from build123d import *

# Parameters (mm, degrees)
BOSS_EXTRUDE1_DEPTH         = 50.8
SKETCH2_R                   = 3.2639
F_1_4_CLEARNACE_HOLES_DEPTH = 9.4996
CUT_EXTRUDE2_REACH          = 75.836
SKETCH3_R                   = 4.7625
SKETCH4_R                   = 4.7625
F_3_8_HEAD_DEPTH            = 5.08


with BuildPart() as part:
    # Sketch1 → Boss-Extrude1 (new body)
    with BuildSketch(Plane(origin=(0, 0, 0), x_dir=(0, 0, -1), z_dir=(1, 0, 0))):
        Polygon((41.796907359, 27.1145), (9.4996, 27.1145), (9.4996, 6.4135), (41.796907359, 6.4135), (41.796907359, 0), (0, 0), (0, 33.528), (41.796907359, 33.528), align=None)
    extrude(amount=BOSS_EXTRUDE1_DEPTH)

    # Sketch2 → 1/4 Clearnace Holes (cut)
    with BuildSketch(Plane(origin=(0, 0, -9.4996), x_dir=(-1, 0, 0), z_dir=(0, 0, -1))):
        with Locations(Location((-38.1, 16.764, 0), (0, 0, 90))):
            Circle(SKETCH2_R)
        with Locations(Location((-12.7, 16.764, 0), (0, 0, 90))):
            Circle(SKETCH2_R)
    extrude(amount=-F_1_4_CLEARNACE_HOLES_DEPTH, mode=Mode.SUBTRACT)

    # Cut-Extrude2: up to this face of the body (flat: up to its plane)
    cut_extrude2_end = Plane(part.part.faces().sort_by_distance((25.4, 33.528, -20.898453679))[0])
    # Sketch3 → Cut-Extrude2 (cut, up to the picked face)
    with BuildSketch(Plane.XZ, mode=Mode.PRIVATE) as cut_extrude2_sk1:
        with Locations(Location((25.4, -25.286907359, 0), (0, 0, 270))):
            Circle(SKETCH3_R)
    cut_extrude2_tool1 = split(extrude(cut_extrude2_sk1.sketch, amount=-CUT_EXTRUDE2_REACH, mode=Mode.PRIVATE), bisect_by=cut_extrude2_end, keep=Keep.BOTH, mode=Mode.PRIVATE)
    # Sketch3 → Cut-Extrude2 (cut, up to the picked face)
    with BuildSketch(Plane.XZ, mode=Mode.PRIVATE) as cut_extrude2_sk2:
        with BuildLine():
            Line((0, -12.7), (13.468510474, -33.146437494))
            ThreePointArc((13.468510474, -33.146437494), (25.4, -39.574407359), (37.331489526, -33.146437494))
            Line((37.331489526, -33.146437494), (50.8, -12.7))
            Line((50.8, -12.7), (50.8, -41.796907359))
            Line((50.8, -41.796907359), (0, -41.796907359))
            Line((0, -41.796907359), (0, -12.7))
        make_face()
    cut_extrude2_tool2 = split(extrude(cut_extrude2_sk2.sketch, amount=-CUT_EXTRUDE2_REACH, mode=Mode.PRIVATE), bisect_by=cut_extrude2_end, keep=Keep.BOTH, mode=Mode.PRIVATE)
    add(cut_extrude2_tool1.solids().sort_by(Axis((25.4, 0, -25.286907), (0, 1, 0)))[0], mode=Mode.SUBTRACT)
    add(cut_extrude2_tool2.solids().sort_by(Axis((6.245364, 0, -23.245262), (0, 1, 0)))[0], mode=Mode.SUBTRACT)

    # Sketch4 → 3/8 Head (cut)
    with BuildSketch(Plane(origin=(0, 0, -9.4996), x_dir=(-1, 0, 0), z_dir=(0, 0, -1))):
        with Locations(Location((-12.7, 16.764, 0), (0, 0, 90))):
            Circle(SKETCH4_R)
        with Locations(Location((-38.1, 16.764, 0), (0, 0, 90))):
            Circle(SKETCH4_R)
    extrude(amount=-F_3_8_HEAD_DEPTH, mode=Mode.SUBTRACT)


solid = part.part
Could you check a few things on this model? Use its own coordinates, in mm. A direction names the side the tool comes from. Coordinates: 2 decimals unless noted, no trailing zeros. Order: outer loops, then holes, each group sorted by start corner. A loop starts at its lowest first (then second) coordinate and runs counter-clockwise, first axis right, second up. Notation, with made-up numbers: (47, -30.75) - (58, -30.75) arc R19 ccw to (58, -21.75) - close; hole circle Ø2 at (36.25, 42.5). An arc over 180 degrees is marked (long way). Answer in a Markdown table with one row per item. Add a question column.
(1) If we section it at A-A, the plane x = 25.4: Please give me the cut outline in (y, z), then the cut area to 3 significant figures.
(2) Will these pins go through, and if not, where does the flat tip stop? pin 1 (3 mm diameter, centred on x = 38.5, y = 16.5, fed in from -Z); pin 2 (6 mm diameter, centred on x = 20.5, y = 13, fed in from -Z); pin 3 (10 mm diameter, centred on x = 19, y = 14.5, fed in from +Z); pin 4 (7.5 mm diameter, centred on x = 12.7, y = 16.764, fed in from -Z).
(3) On a 3-axis mill with a long thin cutter (end or side, diameter ignored), from which of +Z, -Z, +X, -X, +Y, -Y can I reach the whole of each face in a straight line? I mean faces 1 (the face through (25.202, 3.162, -39.573)), 2 (the face through (9.802, 12.985, -6.995)), 3 (the face through (25, 17, -9.5)). Say none if no direction works.
(4) I need wall thicknesses on L1, parallel to Y at x = 21, z = -30.5; L2, parallel to X at y = 12.5, z = -7; L3, parallel to Z at x = 36.5, y = 9. Which ranges of each line are inside material? Lowest first, please.
(5) If we section it at B-B, the plane z = -17.5: Please give me the cut outline in (x, y).
(6) If we mould it in two halves opening along Y, with no side actions, what happens to faces 4 (the face through (28.62, 3.16, -21.78)), 5 (the face through (25, 0, -16)), 6 (the face through (14, 20, -4.42))? For each: released by +Y, released by -Y, zero draft, split by the parting line, or undercut.
(7) If we section it at D-D, the plane z = -28: Please give me the cut outline in (x, y).
(8) If we section it at C-C, the plane y = 17: Please give me the cut outline in (x, z), then the cut area to 3 significant figures.
Results are:
| question | item | result |
|---|---|---|
| 1 | outline | (0, -39.57) - (6.41, -39.57) - (6.41, -30.05) - (0, -30.05) - close; (0, -20.52) - (6.41, -20.52) - (6.41, -9.5) - (27.11, -9.5) - (27.11, -20.52) - (33.53, -20.52) - (33.53, 0) - (0, 0) - close; (27.11, -39.57) - (33.53, -39.57) - (33.53, -30.05) - (27.11, -30.05) - close |
| 1 | area | 582 mm2 |
| 2 | pin 1 | passes through |
| 2 | pin 2 | stops at z = -9.5 |
| 2 | pin 3 | stops at z = 0 |
| 2 | pin 4 | stops at z = -4.42 |
| 3 | face 1 | -Z, +Y, -Y |
| 3 | face 2 | -Z |
| 3 | face 3 | -Z, +X, -X |
| 4 | L1 | y = 0 to 6.41, 27.11 to 33.53 |
| 4 | L2 | x = 0 to 10.58, 14.82 to 35.98, 40.22 to 50.8 |
| 4 | L3 | z = -9.5 to 0 |
| 5 | outline | (3.16, 0) - (47.64, 0) - (47.64, 6.41) - (3.16, 6.41) - close; (3.16, 27.11) - (47.64, 27.11) - (47.64, 33.53) - (3.16, 33.53) - close |
| 6 | face 4 | zero draft |
| 6 | face 5 | released by -Y |
| 6 | face 6 | undercut |
| 7 | outline | (10.08, 0) - (21.49, 0) - (21.49, 6.41) - (10.08, 6.41) - close; (10.08, 27.11) - (21.49, 27.11) - (21.49, 33.53) - (10.08, 33.53) - close; (29.31, 0) - (40.72, 0) - (40.72, 6.41) - (29.31, 6.41) - close; (29.31, 27.11) - (40.72, 27.11) - (40.72, 33.53) - (29.31, 33.53) - close |
| 8 | outline | (0, -9.5) - (7.94, -9.5) - (7.94, -4.42) - (9.44, -4.42) - (9.44, 0) - (0, 0) - close; (15.96, -4.42) - (17.46, -4.42) - (17.46, -9.5) - (33.34, -9.5) - (33.34, -4.42) - (34.84, -4.42) - (34.84, 0) - (15.96, 0) - close; (41.36, -4.42) - (42.86, -4.42) - (42.86, -9.5) - (50.8, -9.5) - (50.8, 0) - (41.36, 0) - close |
| 8 | area | 328 mm2 |
